from build123d import *

# Parameters (mm, degrees)
BOSS_EXTRUDE1_DEPTH            = 15
CUT_EXTRUDE1_REACH             = 17
SKETCH2_R                      = 8
CUT_EXTRUDE2_REACH             = 17
SKETCH3_R                      = 10
F_5_5_5_5_DIAMETER_HOLE1_D     = 5.5
F_5_5_5_5_DIAMETER_HOLE1_DEPTH = 12
CUT_EXTRUDE3_REACH             = 17
CUT_EXTRUDE4_REACH             = 17
F_5_5_5_5_DIAMETER_HOLE2_D     = 5.5
F_5_5_5_5_DIAMETER_HOLE2_DEPTH = 14.9
F_5_5_5_5_DIAMETER_HOLE3_D     = 5.5
F_5_5_5_5_DIAMETER_HOLE3_DEPTH = 18.9
M5_TAPPED_HOLE2_D              = 4.2
M5_TAPPED_HOLE2_DEPTH          = 14
M5_TAPPED_HOLE2_TIP            = 1.2618073
CHAMFER1_SIZE                  = 1
CHAMFER2_SIZE                  = 1
CHAMFER3_SIZE                  = 1
FILLET1_R                      = 1
F_5_5_5_5_DIAMETER_HOLE4_D     = 5.5


with BuildPart() as part:
    # Sketch1 → Boss-Extrude1 (new body)
    with BuildSketch(Plane.XY):
        Polygon((82, 0), (-82, 0), (-82, 12), (-71, 12), (-71, 47), (71, 47), (71, 12), (82, 12), align=None)
    extrude(amount=BOSS_EXTRUDE1_DEPTH)

    # Sketch2 → Cut-Extrude1 (cut, up to next)
    with BuildSketch(Plane.XY.offset(15), mode=Mode.PRIVATE) as cut_extrude1_sk1:
        with Locations((0, 27)):
            Circle(SKETCH2_R)
    cut_extrude1_tool1 = extrude(cut_extrude1_sk1.sketch, amount=-CUT_EXTRUDE1_REACH, mode=Mode.PRIVATE) & part.part
    add(cut_extrude1_tool1.solids().sort_by_distance((0, 27, 15))[0], mode=Mode.SUBTRACT)

    # Sketch3 → Cut-Extrude2 (cut, up to next)
    with BuildSketch(Plane(origin=(0, 0, 0), x_dir=(-1, 0, 0), z_dir=(0, 0, -1)), mode=Mode.PRIVATE) as cut_extrude2_sk1:
        with Locations((-55, 31)):
            Circle(SKETCH3_R)
    cut_extrude2_tool1 = extrude(cut_extrude2_sk1.sketch, amount=-CUT_EXTRUDE2_REACH, mode=Mode.PRIVATE) & part.part
    add(cut_extrude2_tool1.solids().sort_by_distance((55, 31, 0))[0], mode=Mode.SUBTRACT)
    # Sketch3 → Cut-Extrude2 (cut, up to next)
    with BuildSketch(Plane(origin=(0, 0, 0), x_dir=(-1, 0, 0), z_dir=(0, 0, -1)), mode=Mode.PRIVATE) as cut_extrude2_sk2:
        with Locations((55, 31)):
            Circle(SKETCH3_R)
    cut_extrude2_tool2 = extrude(cut_extrude2_sk2.sketch, amount=-CUT_EXTRUDE2_REACH, mode=Mode.PRIVATE) & part.part
    add(cut_extrude2_tool2.solids().sort_by_distance((-55, 31, 0))[0], mode=Mode.SUBTRACT)

    # Ø5.5 (5.5) Diameter Hole1
    with Locations(Plane(origin=(-77, 12, 7.5), x_dir=(0, 0, 1), z_dir=(0, 1, 0))):
        with Locations((0, 0), (0, 154)):
            Hole(F_5_5_5_5_DIAMETER_HOLE1_D / 2, depth=F_5_5_5_5_DIAMETER_HOLE1_DEPTH)

    # Sketch9 → Cut-Extrude3 (cut, up to next)
    with BuildSketch(Plane.XY.offset(15), mode=Mode.PRIVATE) as cut_extrude3_sk1:
        Polygon((0, 41), (-14, 41), (-14, 12), (-35, 12), (-35, 47), (35, 47), (35, 12), (18, 12), (18, 41), align=None)
    cut_extrude3_tool1 = extrude(cut_extrude3_sk1.sketch, amount=-CUT_EXTRUDE3_REACH, mode=Mode.PRIVATE) & part.part
    add(cut_extrude3_tool1.solids().sort_by_distance((-7, 41.782624, 15))[0], mode=Mode.SUBTRACT)

    # Sketch10 → Cut-Extrude4 (cut, up to next)
    with BuildSketch(Plane.XY.offset(15), mode=Mode.PRIVATE) as cut_extrude4_sk1:
        Polygon((-55, 31), (-55, 32.1), (-35, 32.1), (-35, 29.9), (-55, 29.9), align=None)
    cut_extrude4_tool1 = extrude(cut_extrude4_sk1.sketch, amount=-CUT_EXTRUDE4_REACH, mode=Mode.PRIVATE) & part.part
    add(cut_extrude4_tool1.solids().sort_by_distance((-45, 31, 15))[0], mode=Mode.SUBTRACT)
    # Sketch10 → Cut-Extrude4 (cut, up to next)
    with BuildSketch(Plane.XY.offset(15), mode=Mode.PRIVATE) as cut_extrude4_sk2:
        Polygon((55, 31), (55, 32.1), (35, 32.1), (35, 29.9), (55, 29.9), align=None)
    cut_extrude4_tool2 = extrude(cut_extrude4_sk2.sketch, amount=-CUT_EXTRUDE4_REACH, mode=Mode.PRIVATE) & part.part
    add(cut_extrude4_tool2.solids().sort_by_distance((45, 31, 15))[0], mode=Mode.SUBTRACT)
    # Sketch10 → Cut-Extrude4 (cut, up to next)
    with BuildSketch(Plane.XY.offset(15), mode=Mode.PRIVATE) as cut_extrude4_sk3:
        Polygon((0, 27), (0, 28.1), (18, 28.1), (18, 25.9), (0, 25.9), align=None)
    cut_extrude4_tool3 = extrude(cut_extrude4_sk3.sketch, amount=-CUT_EXTRUDE4_REACH, mode=Mode.PRIVATE) & part.part
    add(cut_extrude4_tool3.solids().sort_by_distance((9, 27, 15))[0], mode=Mode.SUBTRACT)

    # Ø5.5 (5.5) Diameter Hole2
    with Locations(Plane(origin=(-40, 47, 7.5), x_dir=(0, 0, 1), z_dir=(0, 1, 0))):
        with Locations((0, 0), (0, 80)):
            Hole(F_5_5_5_5_DIAMETER_HOLE2_D / 2, depth=F_5_5_5_5_DIAMETER_HOLE2_DEPTH)

    # Ø5.5 (5.5) Diameter Hole3
    with Locations(Plane(origin=(13, 47, 7.5), x_dir=(0, 0, 1), z_dir=(0, 1, 0))):
        with Locations((0, 0)):
            Hole(F_5_5_5_5_DIAMETER_HOLE3_D / 2, depth=F_5_5_5_5_DIAMETER_HOLE3_DEPTH)

    # M5 Tapped Hole2
    with Locations(Plane(origin=(-40, 29.9, 7.5), x_dir=(0, 0, 1), z_dir=(0, 1, 0))):
        with Locations((0, 0), (0, 80)):
            Hole(M5_TAPPED_HOLE2_D / 2, depth=M5_TAPPED_HOLE2_DEPTH)
            with Locations((0, 0, -(M5_TAPPED_HOLE2_DEPTH + M5_TAPPED_HOLE2_TIP / 2))):  # 118° drill point
                Cone(0, M5_TAPPED_HOLE2_D / 2, M5_TAPPED_HOLE2_TIP, mode=Mode.SUBTRACT)

    # Chamfer1
    chamfer1_edges = [part.edges().sort_by_distance(p)[0] for p in [
        (-71, 47, 7.5),
        (71, 47, 7.5),
    ]]
    chamfer(chamfer1_edges, length=CHAMFER1_SIZE)

    # Chamfer2
    chamfer2_edges = [part.edges().sort_by_distance(p)[0] for p in [
        (-14, 41, 7.5),
    ]]
    chamfer(chamfer2_edges, length=CHAMFER2_SIZE)

    # Chamfer3
    chamfer3_edges = [part.edges().sort_by_distance(p)[0] for p in [
        (-14, 12, 7.5),
        (-35, 12, 7.5),
        (35, 12, 7.5),
        (18, 12, 7.5),
    ]]
    chamfer(chamfer3_edges, length=CHAMFER3_SIZE)

    # Fillet1
    fillet1_edges = [part.edges().sort_by_distance(p)[0] for p in [
        (35, 29.9, 7.5),
        (35, 32.1, 7.5),
        (45.060684128, 29.9, 7.5),
        (45.060684128, 32.1, 7.5),
        (18, 28.1, 7.5),
        (18, 25.9, 7.5),
        (7.924014134, 28.1, 7.5),
        (7.924014134, 25.9, 7.5),
        (71, 12, 7.5),
        (82, 12, 7.5),
        (-82, 12, 7.5),
        (-71, 12, 7.5),
        (-71, 46, 7.5),
        (-70, 47, 7.5),
        (70, 47, 7.5),
        (71, 46, 7.5),
        (-13, 41, 7.5),
        (-14, 40, 7.5),
        (35, 13, 7.5),
        (19, 12, 7.5),
        (34, 12, 7.5),
        (18, 13, 7.5),
        (-14, 13, 7.5),
        (-34, 12, 7.5),
        (-15, 12, 7.5),
        (-35, 13, 7.5),
        (18, 41, 7.5),
        (-35, 47, 7.5),
        (35, 47, 7.5),
        (-45.060684128, 32.1, 7.5),
        (-45.060684128, 29.9, 7.5),
        (-35, 32.1, 7.5),
        (-35, 29.9, 7.5),
    ]]
    fillet(fillet1_edges, radius=FILLET1_R)

    # Ø5.5 (5.5) Diameter Hole4 (through all)
    with Locations(Plane(origin=(-25, 12, 7.5), x_dir=(1, 0, 0), z_dir=(0, 1, 0))):
        with Locations((0, 0), (50, 0)):
            Hole(F_5_5_5_5_DIAMETER_HOLE4_D / 2)


solid = part.part
Work out the finished part from the listing and answer in its coordinate system (mm). A direction names the side the tool comes from. Give positions to 0.01 mm unless a question says otherwise; leave off trailing zeros. Loops run counter-clockwise (first coordinate to the right, second up) from the corner with the lowest first, then second, coordinate; pieces in that order, holes last. Notation, with made-up numbers: (-14.5, 63) -> (43.5, 63) arc R32 cw to (43.5, 101) -> close; hole circle Ø1 at (-0.5, 34). An arc over 180 degrees is marked (long way). Use a Markdown table: item, result. Add a question column.
1. Find the intervals of material crossed by probe 1 along X at (y, z) = (15.5, 4.5); probe 2 along X at (y, z) = (38.5, 12.5); probe 3 along Y at (x, z) = (0, 8), in increasing order.
2. Section B-B on x = 55 is taken. Determine the outline of the cut face in (y, z), and give its area (3 significant figures).
3. Flat-ended cylindrical pins translate along their axes: pin 1 Ø7.5 at (y, z) = (31, 6) entering from -X; pin 2 Ø7 at (x, z) = (-76.5, 6.5) entering from +Y; pin 3 Ø1.5 at (x, y) = (-32.5, 42) entering from -Z; pin 4 Ø8.5 at (y, z) = (37, 8) entering from +X. Find the tip coordinate at first contact, or state that the pin passes through.
4. For faces 4 (the flat face through (82, 6, 7)), 5 (the flat face through (-22, 12, 6)), 6 (the cylindrical face through (42.727, 39.446, 7.858)), 7 (the flat face through (10, 28.1, 8)), determine the directions among +Z, -Z, +X, -X, +Y, -Y from which every point of the face is accessible in a straight line to the end or side of a thin tool.
5. Section A-A on y = 37 is taken. Determine the outline of the cut face in (x, z).
6. Determine the mould class of faces 1 (the flat face through (1.1, 18.6, 0)), 2 (the flat face through (-71, 29, 7)), 3 (the flat face through (-43, 32.1, 8)) for opening direction X: released by +X, released by -X, zero draft, split by the parting line, or undercut.
7. Section C-C on x = 77 is taken. Determine the outline of the cut face in (y, z), and give its area (3 significant figures).
Results below:
| question | item | result |
|---|---|---|
| 1 | probe 1 | x = -71 to -35, -14 to 18, 35 to 71 |
| 1 | probe 2 | x = -71 to -61.61, -48.39 to -35, -14 to 18, 35 to 48.39, 61.61 to 71 |
| 1 | probe 3 | y = 0 to 19, 35 to 41 |
| 2 | outline | (0, 0) -> (21, 0) -> (21, 15) -> (0, 15) -> close; (41, 0) -> (47, 0) -> (47, 15) -> (41, 15) -> close |
| 2 | area | 405 mm^2 |
| 3 | pin 1 | stops at x = -71 |
| 3 | pin 2 | stops at y = 12 |
| 3 | pin 3 | passes through |
| 3 | pin 4 | stops at x = 71 |
| 4 | face 4 | +Z, -Z, +X, +Y, -Y |
| 4 | face 5 | +Z, -Z, +Y |
| 4 | face 6 | +Y |
| 4 | face 7 | +Z, -Z |
| 5 | outline | (-71, 0) -> (-63, 0) -> (-63, 15) -> (-71, 15) -> close; (-47, 0) -> (-35, 0) -> (-35, 15) -> (-47, 15) -> close; (-14, 0) -> (18, 0) -> (18, 15) -> (-14, 15) -> close; (35, 0) -> (47, 0) -> (47, 15) -> (35, 15) -> close; (63, 0) -> (71, 0) -> (71, 15) -> (63, 15) -> close; hole circle Ø5.5 at (-40, 7.5); hole circle Ø5.5 at (13, 7.5); hole circle Ø5.5 at (40, 7.5) |
| 6 | face 1 | zero draft |
| 6 | face 2 | released by -X |
| 6 | face 3 | undercut |
| 7 | outline | (0, 0) -> (12, 0) -> (12, 4.75) -> (0, 4.75) -> close; (0, 10.25) -> (12, 10.25) -> (12, 15) -> (0, 15) -> close |
| 7 | area | 114 mm^2 |
